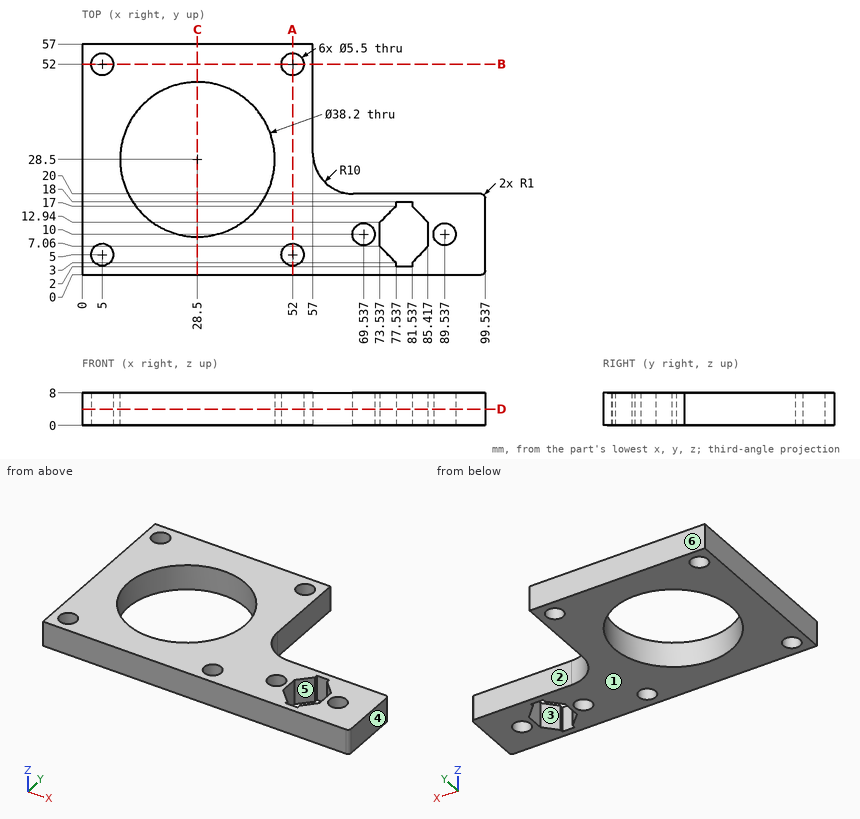
Check sheet for the drawn part. Datum: minimum x, y, z corner. Units: mm. A direction names the side the tool comes from. Round coordinates to 2 decimals unless told otherwise and drop trailing zeros. Loops run counter-clockwise (first coordinate to the right, second up) from the corner with the lowest first, then second, coordinate; pieces in that order, holes last. Notation, with made-up numbers: (5, 15) - (55, 15) arc R12 cw to (55, 23) - close; hole circle Ø11 at (49.25, -28). An arc over 180 degrees is marked (long way). Answer as a JSON object with one key per item and string values. Group by question number.
Q1. Sectioned sample at A-A, the plane x = 52. Enter the section's corners in (y, z), plus the area to 3 significant figures.
Q2. Gauge pin test, flat ends, axial feed: P1, Ø3.5, axis at x = 89.54, y = 10, coming from the +Z side; P2, Ø1.2, axis at x = 80.5, z = 5.5, coming from the +Y side. Record the tip position at first contact, or that the pin passes through.
Q3. Scan lines: line 1 along Y through (x, z) = (52, 6); line 2 along X through (y, z) = (54, 7); line 3 along Y through (x, z) = (28.5, 1.75). Record each from-to range of solid material in increasing order. Write a range as [from, to].
Q4. Sectioned sample at D-D, the plane z = 4. Count the separate pieces of the cut face and the enclosed holes in it, plus the area to 3 significant figures.
Q5. Sectioned sample at C-C, the plane x = 28.5. Enter the section's corners in (y, z).
Q6. Set-up check for the marked faces 1 and 2: record each of +Z, -Z, +X, -X, +Y, -Y from which the full face is reachable in a straight line by a thin tool's end or side.
Q7. Mould release check, pull along X, two halves, no side actions. Record for the marked faces 3, 4, 5 and 6: released by +X, released by -X, zero draft, split by the parting line, or undercut.
Solution:
{
 "1": {"outline": "(0, 0) - (2.25, 0) - (2.25, 8) - (0, 8) - close; (7.75, 0) - (49.25, 0) - (49.25, 8) - (7.75, 8) - close; (54.75, 0) - (57, 0) - (57, 8) - (54.75, 8) - close", "area": "368 mm²"},
 "2": {"P1": "passes through", "P2": "stops at y = 20"},
 "3": {"line 1": "y = [0, 2.25], [7.75, 49.25], [54.75, 57]", "line 2": "x = [0, 3.11], [6.89, 50.11], [53.89, 57]", "line 3": "y = [0, 9.4], [47.6, 57]"},
 "4": {"separate pieces": "1", "enclosed holes": "8", "area": "2,690 mm²"},
 "5": {"outline": "(0, 0) - (9.4, 0) - (9.4, 8) - (0, 8) - close; (47.6, 0) - (57, 0) - (57, 8) - (47.6, 8) - close"},
 "6": {"face 1": "-Z, +X, -X, +Y, -Y", "face 2": "+Z, -Z, +X, +Y"},
 "7": {"face 3": "undercut", "face 4": "released by +X", "face 5": "undercut", "face 6": "zero draft"}
}
